Geometry: final body of the model. Coordinates: model frame, mm. Face numbers are marked on the shaded views. Round coordinates to 2 decimals unless told otherwise and drop trailing zeros. Order: outer loops, then holes, each group sorted by start corner. A loop starts at its lowest first (then second) coordinate and runs counter-clockwise, first axis right, second up. Notation, with made-up numbers: (-4.75, 80.5) - (34.25, 80.5) arc R17 ccw to (34.25, 98.5) - close; hole circle Ø8 at (54.5, 36). An arc over 180 degrees is marked (long way). Put each result on its own line as item: value. Start each with the question number.
(1) Section C-C (y = 1). Output: boundary loops of the cut face in (x, z) (3 decimals), and give its area (3 significant figures).
(2) Section A-A (x = 16). Output: boundary loops of the cut face in (y, z) (3 decimals).
(3) Section D-D (z = 18.5). Output: boundary loops of the cut face in (x, y) (3 decimals).
(4) Pin query (flat end, axial travel): P1, Ø1.6, axis at x = -43.5, z = 12.5, coming from the +Y side; P2, Ø0.8, axis at x = -41, y = 3.5, coming from the -Z side; P3, Ø8, axis at x = 10.5, z = 21, coming from the -Y side; P4, Ø2, axis at x = 43.5, y = 2.5, coming from the -Z side. Return the tip coordinate at first contact, or that it passes through.
(5) Section B-B (y = 5). Count the separate pieces of the cut face and the enclosed holes in it, and give its area (3 significant figures).
(6) Pull-direction query (X, two-part tool) for the marked faces 1, 2 and 3; classes: released by +X, released by -X, zero draft, split by the parting line, or undercut.
(7) Material intervals for L1, parallel to Z at x = -29.5, y = 4.5 (3 decimals); L2, parallel to X at y = 2, z = 20.5 (3 decimals); L3, parallel to Z at x = 39, y = 2.5, sorted ascending. Write a range as [from, to].
from build123d import *

# Parameters (mm, degrees)
BOSS_EXTRUDE3_DEPTH = 6.35
ANTENNA_HOLE_SIZE_W = 7
ANTENNA_HOLE_SIZE_H = 6
CUT_EXTRUDE3_DEPTH  = 3.175
SKETCH7_R           = 1.4732
CUT_EXTRUDE4_DEPTH  = 10
SKETCH8_W           = 3.175
SKETCH8_H           = 43.3
CUT_EXTRUDE5_DEPTH  = 55.454774814


with BuildPart() as part:
    # Sketch2 → Boss-Extrude3 (new body)
    with BuildSketch(Plane(origin=(0, 0, 0), x_dir=(1, 0, 0), z_dir=(0, 1, 0))):
        with BuildLine():
            Line((-45, 25.825), (-45, -25.825))
            ThreePointArc((-45, -25.825), (-43.777170811, -28.777170811), (-40.825, -30))
            Line((-40.825, -30), (40.825, -30))
            ThreePointArc((40.825, -30), (43.777170811, -28.777170811), (45, -25.825))
            Line((45, -25.825), (45, 25.825))
            ThreePointArc((45, 25.825), (43.777170811, 28.777170811), (40.825, 30))
            Line((40.825, 30), (-40.825, 30))
            ThreePointArc((-40.825, 30), (-43.777170811, 28.777170811), (-45, 25.825))
        make_face()
        with BuildLine():
            Line((40.825, 21.65), (41.825, 21.65))
            Line((41.825, 21.65), (41.825, -21.65))
            Line((41.825, -21.65), (40.825, -21.65))
            ThreePointArc((40.825, -21.65), (37.872829189, -22.872829189), (36.65, -25.825))
            Line((36.65, -25.825), (36.65, -26.825))
            Line((36.65, -26.825), (-36.65, -26.825))
            Line((-36.65, -26.825), (-36.65, -25.825))
            ThreePointArc((-36.65, -25.825), (-37.872829189, -22.872829189), (-40.825, -21.65))
            Line((-40.825, -21.65), (-41.825, -21.65))
            Line((-41.825, -21.65), (-41.825, 21.65))
            Line((-41.825, 21.65), (-40.825, 21.65))
            ThreePointArc((-40.825, 21.65), (-37.872829189, 22.872829189), (-36.65, 25.825))
            Line((-36.65, 25.825), (-36.65, 26.825))
            Line((-36.65, 26.825), (36.65, 26.825))
            Line((36.65, 26.825), (36.65, 25.825))
            ThreePointArc((36.65, 25.825), (37.872829189, 22.872829189), (40.825, 21.65))
        make_face(mode=Mode.SUBTRACT)
    extrude(amount=BOSS_EXTRUDE3_DEPTH)

    # Antenna Hole Size → Cut-Extrude3 (cut)
    with BuildSketch(Plane.ZY.offset(45)):
        with Locations((13.825, 6.35)):
            Rectangle(ANTENNA_HOLE_SIZE_W, ANTENNA_HOLE_SIZE_H)
    extrude(amount=-CUT_EXTRUDE3_DEPTH, mode=Mode.SUBTRACT)

    # Sketch7 → Cut-Extrude4 (cut)
    with BuildSketch(Plane.XZ):
        with Locations(Location((-40.825, -25.825, 0), (0, 0, 270))):
            Circle(SKETCH7_R)
        with Locations(Location((-40.825, 25.825, 0), (0, 0, 270))):
            Circle(SKETCH7_R)
        with Locations(Location((40.825, 25.825, 0), (0, 0, 270))):
            Circle(SKETCH7_R)
        with Locations(Location((40.825, -25.825, 0), (0, 0, 270))):
            Circle(SKETCH7_R)
    extrude(amount=-CUT_EXTRUDE4_DEPTH, mode=Mode.SUBTRACT)

    # Sketch8 → Cut-Extrude5 (cut, through all)
    with BuildSketch(Plane(origin=(0, 6.35, 0), x_dir=(1, 0, 0), z_dir=(0, 1, 0))):
        with Locations((43.4125, 0)):
            Rectangle(SKETCH8_W, SKETCH8_H)
    extrude(amount=-CUT_EXTRUDE5_DEPTH, mode=Mode.SUBTRACT)


solid = part.part
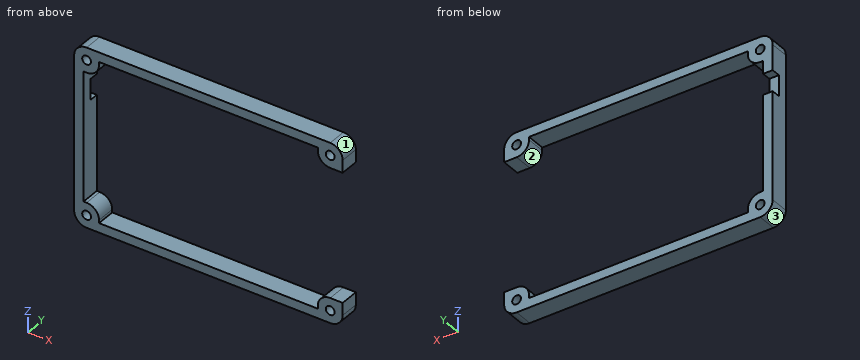
Checks:
1. outline: (-45, -25.825) arc R4.175 ccw to (-40.825, -30) - (40.825, -30) arc R4.175 ccw to (45, -25.825) - (45, -21.65) - (40.825, -21.65) arc R4.175 ccw to (36.65, -25.825) - (36.65, -26.825) - (-36.65, -26.825) - (-36.65, -25.825) arc R4.175 ccw to (-40.825, -21.65) - (-41.825, -21.65) - (-41.825, 21.65) - (-40.825, 21.65) arc R4.175 ccw to (-36.65, 25.825) - (-36.65, 26.825) - (36.65, 26.825) - (36.65, 25.825) arc R4.175 ccw to (40.825, 21.65) - (45, 21.65) - (45, 25.825) arc R4.175 ccw to (40.825, 30) - (-40.825, 30) arc R4.175 ccw to (-45, 25.825) - close; hole circle Ø2.946 at (-40.825, -25.825); hole circle Ø2.946 at (-40.825, 25.825); hole circle Ø2.946 at (40.825, -25.825); hole circle Ø2.946 at (40.825, 25.825)
1. area: 825 mm²
2. outline: (0, -30) - (6.35, -30) - (6.35, -26.825) - (0, -26.825) - close; (0, 26.825) - (6.35, 26.825) - (6.35, 30) - (0, 30) - close
3. outline: (-45, 0) - (-41.825, 0) - (-41.825, 6.35) - (-45, 6.35) - close
4. P1: stops at y = 3.35
4. P2: stops at z = -30
4. P3: passes through
4. P4: stops at z = -29.65
5. separate pieces: 2
5. enclosed holes: 4
5. area: 802 mm²
6. face 1: released by +X
6. face 2: undercut
6. face 3: released by -X
7. L1: z = [-30, -26.825], [26.825, 30]
7. L2: x = [-45, -41.825]
7. L3: z = [-30, -22.07], [22.07, 30]
